Design review of the part built by this model. Coordinates are the model's own, in mm. A direction names the side the tool comes from. Coordinates: 2 decimals unless noted, no trailing zeros. Loops run counter-clockwise (first coordinate to the right, second up) from the corner with the lowest first, then second, coordinate; pieces in that order, holes last. Notation, with made-up numbers: (-39.5, 62.25) -> (-30.5, 62.25) arc R24 ccw to (-30.5, 90.25) -> close; hole circle Ø4 at (66.5, 63). An arc over 180 degrees is marked (long way). Answer as a JSON object with one key per item and string values.
```python
from build123d import *

# Parameters (mm, degrees)
PAD_DEPTH     = 15
SKETCH001_R   = 9.75
SKETCH001_R_2 = 8.25
PAD001_DEPTH  = 7.8
FILLET_R      = 2


with BuildPart() as part:
    # Sketch → Pad (new body)
    with BuildSketch(Plane.XZ):
        with BuildLine():
            ThreePointArc((3.68273, 0), (0, 7.75), (-3.68273, 0))
            Line((-3.68273, 0), (3.68273, 0))
        make_face()
    extrude(amount=PAD_DEPTH)

    # Sketch001 → Pad001 (join)
    with BuildSketch(Plane.XY):
        with Locations((0, 9.75)):
            Circle(SKETCH001_R)
        with Locations((0, 9.75)):
            Circle(SKETCH001_R_2, mode=Mode.SUBTRACT)
        Polygon((-4.75, 0), (-4.75, 1.235307), (0, 0), (4.75, 1.235307), (4.75, 0), align=None)
    extrude(amount=PAD001_DEPTH)

    # Fillet
    fillet_edges = [part.edges().sort_by_distance(p)[0] for p in [
        (0, -15, 7.75),
        (0, -15, 0),
    ]]
    fillet(fillet_edges, radius=FILLET_R)


solid = part.part
```
1) Add section A-A, the plane x = 0. Give the boundary of the cut face in (y, z), and give its area (3 significant figures).
Completed:
{"outline": "(-15, 2) arc R2 ccw to (-13, 0) -> (1.5, 0) -> (1.5, 7.8) -> (0, 7.8) -> (0, 7.75) -> (-13, 7.75) arc R2 ccw to (-15, 5.75) -> close; (18, 0) -> (19.5, 0) -> (19.5, 7.8) -> (18, 7.8) -> close", "area": "138 mm²"}
2) Add section B-B, the plane y = 9.75. Give the boundary of the cut face in (x, z), and give its area (3 significant figures).
Completed:
{"outline": "(-9.75, 0) -> (-8.25, 0) -> (-8.25, 7.8) -> (-9.75, 7.8) -> close; (8.25, 0) -> (9.75, 0) -> (9.75, 7.8) -> (8.25, 7.8) -> close", "area": "23.4 mm²"}
3) Add section D-D, the plane y = 17.5. Give the boundary of the cut face in (x, z).
Completed:
{"outline": "(-5.92, 0) -> (-2.83, 0) -> (-2.83, 7.8) -> (-5.92, 7.8) -> close; (2.83, 0) -> (5.92, 0) -> (5.92, 7.8) -> (2.83, 7.8) -> close"}
4) Add section C-C, the plane y = -0.5. Give the boundary of the cut face in (x, z), and give its area (3 significant figures).
Completed:
{"outline": "(-3.68, 0) -> (3.68, 0) arc R4.75 ccw (long way) to start", "area": "61.9 mm²"}
5) The part is to be moulded in two halves that separate along Y. For faces 1 (the cylindrical face through (0.05, -14.4, 0.57)), 2 (the cylindrical face through (-1.8, 1.7, 3.8)), 3 (the flat face through (1, 1, 0)), say which applies: pulls with the +Y half, pulls with the -Y half, needs draft (parallel to the pull), parting line crosses it, or undercut.
Completed:
{"face 1": "pulls with the -Y half", "face 2": "undercut", "face 3": "needs draft"}
6) Clearance check with flat-ended pins moving along their axes: pin 1 Ø6 at (x, y) = (1.5, -5.5) entering from +Z; pin 2 Ø1.4 at (x, z) = (2, 6) entering from -Y; pin 3 Ø2 at (y, z) = (5, 6) entering from -X; pin 4 Ø1.5 at (x, y) = (-6, 6) entering from -Z (3 decimals). State where each tip first meets the part, or that it passes through.
Completed:
{"pin 1": "z = 7.75", "pin 2": "y = -14.99", "pin 3": "x = -9", "pin 4": "through"}
7) For faces 4 (the cylindrical face through (0.15, -6.409, 7.748)), 5 (the flat face through (-4.5, 0, 0.7)), 6 (the flat face through (-4.75, 1, 4)), 7 (the flat face through (4.75, 1, 4)), 8 (the flat face through (4.4, 0, 0.8)), list the 3-axis set-ups (+Z, -Z, +X, -X, +Y, -Y) from which the entire face can be reached by the end or side of a thin tool; tool diameter is ignored.
Completed:
{"face 4": "-Y", "face 5": "-Z, -X, -Y", "face 6": "+Z, -Z, -X, -Y", "face 7": "+Z, -Z, +X, -Y", "face 8": "-Z, +X, -Y"}
8) Wall thickness on probe 1 along Y at (x, z) = (0, 2.5); probe 2 along Y at (x, z) = (-6.75, 2.75); probe 3 along X at (y, z) = (5.5, 5.5): over which ranges is each line inside the solid? List them lowest first.
Completed:
{"probe 1": "-15 to 1.5, 18 to 19.5", "probe 2": "2.71 to 5.01, 14.49 to 16.79", "probe 3": "-8.77 to -7.07, 7.07 to 8.77"}
